```python
from build123d import *

# Parameters (mm, degrees)
F0_W     = 101.6
F0_H     = 101.6
F1_DEPTH = 3.175
F3_DEPTH = 3.176
F5_DEPTH = 25.4


with BuildPart() as f1:
    # F0 (on Front) → F1 (new body)
    with BuildSketch(Plane.XZ):
        Rectangle(F0_W, F0_H)
    extrude(amount=F1_DEPTH)

    # F2 (on face) → F3 (cut, through all)
    with BuildSketch(Plane.XZ.offset(3.175)):
        Polygon((32.6009, 50.8), (-32.6009, 50.8), (0, 20.584378), align=None)
    extrude(amount=-F3_DEPTH, mode=Mode.SUBTRACT)

    # F4 (on face) → F5 (cut)
    with BuildSketch(Plane.XZ.offset(3.175)):
        Polygon((0, -8.143783), (-42.656217, -50.8), (42.656217, -50.8), align=None)
    extrude(amount=-F5_DEPTH, mode=Mode.SUBTRACT)


solid = f1.part
```
The listing builds one solid part. Answer for the finished solid, in the listing's coordinates (mm). A direction names the side the tool comes from. Coordinates: 2 decimals unless noted, no trailing zeros. Loops run counter-clockwise (first coordinate to the right, second up) from the corner with the lowest first, then second, coordinate; pieces in that order, holes last. Notation, with made-up numbers: M 77,-19 L 90,-19 A7 cw 90,-13 Z; hole C -20,-0.5 d9. An arc over 180 degrees is marked long. Answer as a JSON object with one key per item and string values. Group by question number.
Item 1: Section B-B (y = -1.9) is taken. Write down the section's boundary in (x, z).
Item 2: Section D-D (x = 30) is taken. Write down the section's boundary in (y, z) (3 decimals), and give its area (3 significant figures).
Item 3: Section A-A (z = -25) is taken. Write down the section's boundary in (x, y) (3 decimals).
Item 4: Section C-C (x = 14) is taken. Write down the section's boundary in (y, z) (3 decimals), and give its area (3 significant figures).
Item 5: Consider L1, parallel to X at y = -2.55, z = -17.5; L2, parallel to X at y = -0.85, z = -33; L3, parallel to Z at x = -12.5, y = -0.15. Determine where each line is inside the solid, lowest interval first.
Item 6: Determine the mould class of faces 4 (the face through (-47, -2, -50.8)), 5 (the face through (50.8, -2, -1)), 6 (the face through (-16.529, -1.61, 35.904)) for opening direction X: +X half, -X half, draft (parallel to the pull), parting line (faces both ways), or undercut.
Item 7: Which of the six approach directions +Z, -Z, +X, -X, +Y, -Y give full straight-line access (tool end or side, diameter ignored) to faces 1 (the face through (21.627, -1.61, -29.77)), 2 (the face through (16.07, -1.61, 35.48)), 3 (the face through (-1, -3.175, 1))?
Item 8: This flat-tipped pin is pushed along its axis until it touches: P1, Ø5, axis at x = -38, z = -8, coming from the +Y side. Where does it stop, or does it pass through?
Solved:
{
 "1": {"outline": "M -50.8,-50.8 L -42.66,-50.8 L 0,-8.14 L 42.66,-50.8 L 50.8,-50.8 L 50.8,50.8 L 32.6,50.8 L 0,20.58 L -32.6,50.8 L -50.8,50.8 Z"},
 "2": {"outline": "M -3.175,-38.144 L 0,-38.144 L 0,48.389 L -3.175,48.389 Z", "area": "275 mm2"},
 "3": {"outline": "M -50.8,-3.175 L -16.856,-3.175 L -16.856,0 L -50.8,0 Z; M 16.856,-3.175 L 50.8,-3.175 L 50.8,0 L 16.856,0 Z"},
 "4": {"outline": "M -3.175,-22.144 L 0,-22.144 L 0,33.56 L -3.175,33.56 Z", "area": "177 mm2"},
 "5": {"L1": "x = -50.8 to -9.36, 9.36 to 50.8", "L2": "x = -50.8 to -24.86, 24.86 to 50.8", "L3": "z = -20.64 to 32.17"},
 "6": {"face 4": "draft", "face 5": "+X half", "face 6": "undercut"},
 "7": {"face 1": "-Z, +Y, -Y", "face 2": "+Z, +Y, -Y", "face 3": "+Z, -Z, +X, -X, -Y"},
 "8": {"P1": "stops at y = 0"}
}
